```python
from build123d import *

# Parameters (mm, degrees)
F1_DEPTH  = 90.5500094
F2_R      = 11.2530001
F2_R_2    = 1.5
F2_R_3    = 2.5
F3_DEPTH  = 1.70942
F4_R      = 1.35255
F5_DEPTH  = 260.59384
F6_R      = 0.762
F7_R      = 1.35255
F8_DEPTH  = 260.59384
F9_W      = 227.80752
F9_H      = 3.69316
F10_DEPTH = 1.70942
F11_W     = 227.80752
F11_H     = 1.70942
F12_DEPTH = 12.5218698
F13_R     = 3.69316
F14_R     = 1.98374
F15_SIZE  = 8.9506298
F16_W     = 6
F16_H     = 1.5875
F17_DEPTH = 97.9363294


with BuildPart() as f1:
    # F0 (on Top) → F1 (new body)
    with BuildSketch(Plane.XY):
        Polygon((0, -30.6212494), (0, 0), (-1.70942, 0), (-1.70942, -32.3306694), (258.88442, -32.3306694), (258.88442, 0), (257.175, 0), (257.175, -30.6212494), align=None)
    extrude(amount=F1_DEPTH)

    # F2 (on face) → F3 (cut, through all)
    with BuildSketch(Plane.XZ.offset(32.3306694)):
        with Locations((23.4867323, 45.2750047)):
            Circle(F2_R)
        with Locations((7.9867379, 29.7750103)):
            Circle(F2_R_2)
        with Locations((38.9867267, 29.7750103)):
            Circle(F2_R_2)
        with Locations((38.9867267, 60.7749991)):
            Circle(F2_R_2)
        with Locations((7.9867379, 60.7749991)):
            Circle(F2_R_2)
        with Locations((236.4749906, 40.4499953)):
            Circle(F2_R_3)
    extrude(amount=-F3_DEPTH, mode=Mode.SUBTRACT)

    # F4 (on face) → F5 (cut, through all)
    with BuildSketch(Plane.YZ.offset(258.88442)):
        with Locations((-7.174992, 18.3187594)):
            Circle(F4_R)
        with Locations((-7.174992, 72.23125)):
            Circle(F4_R)
    extrude(amount=-F5_DEPTH, mode=Mode.SUBTRACT)

    # F6
    f6_edges = [f1.edges().sort_by_distance(p)[0] for p in [
        (258.02971, 0, 90.550009),
        (258.02971, 0, 0),
        (-0.85471, 0, 90.550009),
        (-0.85471, 0, 0),
    ]]
    fillet(f6_edges, radius=F6_R)

    # F7 (on face) → F8 (cut, through all)
    with BuildSketch(Plane.YZ.offset(258.88442)):
        with Locations((-24.6687594, 27.9687528)):
            Circle(F7_R)
        with Locations((-3.96875, 27.9687528)):
            Circle(F7_R)
        with Locations((-3.96875, 62.5812566)):
            Circle(F7_R)
        with Locations((-24.6687594, 62.5812566)):
            Circle(F7_R)
    extrude(amount=-F8_DEPTH, mode=Mode.SUBTRACT)

    # F9 (on face) → F10 (join, through all)
    with BuildSketch(Plane(origin=(0, -30.6212494, 0), x_dir=(-1, 0, 0), z_dir=(0, 1, 0))):
        with Locations((-128.5875, -1.84658)):
            Rectangle(F9_W, F9_H)
        with Locations((-128.5875, 92.3965894)):
            Rectangle(F9_W, F9_H)
    extrude(amount=-F10_DEPTH)

    # F11 (on face) → F12 (join)
    with BuildSketch(Plane(origin=(0, -30.6212494, 0), x_dir=(-1, 0, 0), z_dir=(0, 1, 0))):
        with Locations((-128.5875, 93.3884594)):
            Rectangle(F11_W, F11_H)
        with Locations((-128.5875, -2.83845)):
            Rectangle(F11_W, F11_H)
    extrude(amount=F12_DEPTH)

    # F13
    f13_edges = [f1.edges().sort_by_distance(p)[0] for p in [
        (-1.70942, -32.330669, 45.275005),
        (258.88442, -32.330669, 45.275005),
        (128.5875, -32.330669, 94.243169),
        (128.5875, -32.330669, -3.69316),
    ]]
    fillet(f13_edges, radius=F13_R)

    # F14
    f14_edges = [f1.edges().sort_by_distance(p)[0] for p in [
        (0, -30.621249, 45.275005),
        (257.175, -30.621249, 45.275005),
        (128.5875, -30.621249, 92.533749),
        (128.5875, -30.621249, -1.98374),
    ]]
    fillet(f14_edges, radius=F14_R)

    # F15
    f15_edges = [f1.edges().sort_by_distance(p)[0] for p in [
        (14.68374, -18.09938, 93.388459),
        (242.49126, -18.09938, 93.388459),
        (242.49126, -18.09938, -2.83845),
        (14.68374, -18.09938, -2.83845),
    ]]
    chamfer(f15_edges, length=F15_SIZE)

    # F16 (on face) → F17 (cut, through all)
    with BuildSketch(Plane(origin=(0, 0, -3.69316), x_dir=(1, 0, 0), z_dir=(0, 0, -1))):
        with Locations((49.5772186, 20.4806296)):
            Rectangle(F16_W, F16_H)
        with Locations((207.5977814, 20.4806296)):
            Rectangle(F16_W, F16_H)
        with Locations((49.5772186, 24.4493796)):
            Rectangle(F16_W, F16_H)
        with Locations((207.5977814, 24.4493796)):
            Rectangle(F16_W, F16_H)
    extrude(amount=-F17_DEPTH, mode=Mode.SUBTRACT)


solid = f1.part
```
Geometry check sheet. Reference: the model listing, model coordinates, mm. A direction names the side the tool comes from. Coordinates: 2 decimals unless noted, no trailing zeros. Loops run counter-clockwise (first coordinate to the right, second up) from the corner with the lowest first, then second, coordinate; pieces in that order, holes last. Notation, with made-up numbers: (0, -21) - (13, -21) arc R17 cw to (13, 10) - close; hole circle Ø11 at (86, 75.25). An arc over 180 degrees is marked (long way). One line per item, written item: value. Start each with the question number.
(1) Material ranges on line 1 (X direction, y = -22.5, z = 14) (3 decimals); line 2 (Z direction, x = 57, y = -26); line 3 (Y direction, x = 158.5, z = 37), recorded low to high. Write a range as [from, to].
(2) Cross-section at A-A on y = -14. Enter the section's corners in (x, z) (3 decimals), plus the area to 3 significant figures.
(3) Cross-section at C-C on z = 4. Enter the section's corners in (x, y) (1 decimal), plus the area to 3 significant figures.
(4) Tool access check on faces 5 (the flat face through (257.175, -14, 45)), 6 (the flat face through (257.33, -19.98, 0)), 7 (the flat face through (-0.2, -20, 0)). Record the directions out of +Z, -Z, +X, -X, +Y, -Y that give a thin tool (end or side, any length) a straight path to the whole face; none if there is none.
(5) Cross-section at B-B on x = 31. Enter the section's corners in (y, z).
(6) Depth check by flat-ended pin: P1, Ø4, axis at x = 91, z = 42, coming from the +Y side; P2, Ø1.4, axis at x = 50, z = 93, coming from the +Y side; P3, Ø1.8, axis at x = 7.99, z = 29.78, coming from the +Y side; P4, Ø1.3, axis at y = -20.5, z = -2.5, coming from the -X side. Enter the tip coordinate at first touch or a pass-through.
(7) Mould release check, pull along Z, two halves, no side actions. Record for faces 1 (the flat face through (130, -23, -3.693)), 2 (the flat face through (130, -23, 94.243)), 3 (the flat face through (0, -15, 45)), 4 (the cylindrical face through (234.49, -31.49, 38.93)): released by +Z, released by -Z, zero draft, split by the parting line, or undercut.
(8) Cross-section at D-D on x = 172.5. Enter the section's corners in (y, z).
Results below:
1. line 1: x = [-1.709, 0], [257.175, 258.884]
1. line 2: z = [-3.69, -1.98], [92.53, 94.24]
1. line 3: y = [-32.33, -30.62]
2. outline: (-1.709, 0) - (0, 0) - (0, 90.55) - (-1.709, 90.55) - close; (257.175, 0) - (258.884, 0) - (258.884, 90.55) - (257.175, 90.55) - close
2. area: 310 mm2
3. outline: (-1.7, -28.6) arc R3.7 ccw to (2, -32.3) - (255.2, -32.3) arc R3.7 ccw to (258.9, -28.6) - (258.9, 0) - (257.2, 0) - (257.2, -28.6) arc R2 cw to (255.2, -30.6) - (2, -30.6) arc R2 cw to (0, -28.6) - (0, 0) - (-1.7, 0) - close
3. area: 546 mm2
4. face 5: +Z, -Z, +Y
4. face 6: -Z, +X, +Y, -Y
4. face 7: -Z, -X, +Y, -Y
5. outline: (-32.33, 0) arc R3.69 ccw to (-28.64, -3.69) - (-18.1, -3.69) - (-18.1, -1.98) - (-28.64, -1.98) arc R1.98 cw to (-30.62, 0) - (-30.62, 36.9) - (-32.33, 36.9) - close; (-32.33, 53.65) - (-30.62, 53.65) - (-30.62, 90.55) arc R1.98 cw to (-28.64, 92.53) - (-18.1, 92.53) - (-18.1, 94.24) - (-28.64, 94.24) arc R3.69 ccw to (-32.33, 90.55) - close
6. P1: stops at y = -30.62
6. P2: stops at y = -18.1
6. P3: passes through
6. P4: stops at x = 20.58
7. face 1: released by -Z
7. face 2: released by +Z
7. face 3: zero draft
7. face 4: undercut
8. outline: (-32.33, 0) arc R3.69 ccw to (-28.64, -3.69) - (-18.1, -3.69) - (-18.1, -1.98) - (-28.64, -1.98) arc R1.98 cw to (-30.62, 0) - (-30.62, 90.55) arc R1.98 cw to (-28.64, 92.53) - (-18.1, 92.53) - (-18.1, 94.24) - (-28.64, 94.24) arc R3.69 ccw to (-32.33, 90.55) - close
